from build123d import *

# Parameters (mm, degrees)
F1_DEPTH = 152.4
F3_DEPTH = 149.225
F5_DEPTH = 25.4


with BuildPart() as f1:
    # F0 (on Top) → F1 (new body)
    with BuildSketch(Plane.XY):
        Polygon((-177.8, 774.7), (-190.5, 0), (190.5, 0), (177.8, 774.7), align=None)
        Polygon((190.5, 0), (-190.5, 0), (0, -31.75), align=None)
    extrude(amount=F1_DEPTH)

    # F2 (on face) → F3 (cut)
    with BuildSketch(Plane(origin=(0, 0, 0), x_dir=(1, 0, 0), z_dir=(0, 0, -1))):
        Polygon((0, 28.5312048277), (-180.9470539995, -1.6266375055), (-168.3257693684, -771.525), (168.3257693684, -771.525), (180.9470539995, -1.6266375055), align=None)
    extrude(amount=-F3_DEPTH, mode=Mode.SUBTRACT)

    # F4 (on face) → F5 (cut)
    with BuildSketch(Plane.XY.offset(152.4)):
        with BuildLine():
            Line((114.3, 717.55), (-114.3, 717.55))
            ThreePointArc((-114.3, 717.55), (-132.2605122421, 710.1105122421), (-139.7, 692.15))
            Line((-139.7, 692.15), (-139.7, 323.85))
            ThreePointArc((-139.7, 323.85), (-132.2605122421, 305.8894877579), (-114.3, 298.45))
            Line((-114.3, 298.45), (114.3, 298.45))
            ThreePointArc((114.3, 298.45), (132.2605122421, 305.8894877579), (139.7, 323.85))
            Line((139.7, 323.85), (139.7, 692.15))
            ThreePointArc((139.7, 692.15), (132.2605122421, 710.1105122421), (114.3, 717.55))
        make_face()
    extrude(amount=-F5_DEPTH, mode=Mode.SUBTRACT)


solid = f1.part
The listing builds one solid part. Answer for the finished solid, in the listing's coordinates (mm). A direction names the side the tool comes from. Round coordinates to 2 decimals unless told otherwise and drop trailing zeros. Loops run counter-clockwise (first coordinate to the right, second up) from the corner with the lowest first, then second, coordinate; pieces in that order, holes last. Notation, with made-up numbers: M -21.75,46.25 L -15.75,46.25 A10 ccw -15.75,56.25 Z; hole C 34.5,-31.5 d6. An arc over 180 degrees is marked long. Write each question's results on one line, items separated by ' | '. Start each with the question number.
1) Find section B-B on x = 12.5. Write down the section's boundary in (y, z) (3 decimals), plus the area to 3 significant figures.
2) Which of the six approach directions +Z, -Z, +X, -X, +Y, -Y give full straight-line access (tool end or side, diameter ignored) to faces 5 (the flat face through (-3, 288, 152.4)), 6 (the flat face through (-2, 771.525, 74)), 7 (the cylindrical face through (-132.46, 306.09, 150.83))?
3) Straight lines are drawn through the part: probe 1 along Y at (x, z) = (-0.5, 111) (3 decimals); probe 2 along X at (y, z) = (416, 100); probe 3 along Y at (x, z) = (77.5, 119) (3 decimals). For each, find the intervals that lie inside material, in ascending order.
4) Find section D-D on x = 154. Write down the section's boundary in (y, z) (3 decimals), plus the area to 3 significant figures.
5) Determine the mould class of faces 1 (the flat face through (-3, 277, 149.225)), 2 (the cylindrical face through (132.06, 305.69, 150.83)), 3 (the flat face through (-96.583, -15.653, 75.133)), 4 (the flat face through (2, 774.7, 75)) for opening direction Y: pulls with the +Y half, pulls with the -Y half, needs draft (parallel to the pull), parting line crosses it, or undercut.
6) Find section C-C on y = 663.5. Write down the section's boundary in (x, z) (3 decimals), plus the area to 3 significant figures.
7) Each of these flat-tipped pins is pushed along its axis until it touches: pin 1 (2.5 mm diameter, centred on y = 514.5, z = 151, fed in from -X); pin 2 (1 mm diameter, centred on x = -43.5, z = 20.5, fed in from -Y); pin 3 (1 mm diameter, centred on y = 485.5, z = 151, fed in from +X). Where does it stop, or does it pass through?
8) Find section A-A on z = 47. Write down the section's boundary in (x, y) (3 decimals), plus the area to 3 significant figures.
Final values:
1) outline: M -29.667,0 L -26.448,0 L -26.448,149.225 L 298.45,149.225 L 298.45,152.4 L -29.667,152.4 Z; M 717.55,149.225 L 771.525,149.225 L 771.525,0 L 774.7,0 L 774.7,152.4 L 717.55,152.4 Z | area: 2,180 mm²
2) face 5: +Z, +X, -X, +Y, -Y | face 6: -Z | face 7: +Z, -Z
3) probe 1: -31.667 to -28.448, 771.525 to 774.7 | probe 2: -183.68 to -174.15, 174.15 to 183.68 | probe 3: -18.833 to -15.615, 771.525 to 774.7
4) outline: M -6.083,0 L -2.865,0 L -2.865,149.225 L 771.525,149.225 L 771.525,0 L 774.7,0 L 774.7,152.4 L -6.083,152.4 Z | area: 3,430 mm²
5) face 1: undercut | face 2: undercut | face 3: pulls with the -Y half | face 4: pulls with the +Y half
6) outline: M -179.623,0 L -170.097,0 L -170.097,149.225 L -139.7,149.225 L -139.7,152.4 L -179.623,152.4 Z; M 139.7,149.225 L 170.097,149.225 L 170.097,0 L 179.623,0 L 179.623,152.4 L 139.7,152.4 Z | area: 3,100 mm²
7) pin 1: x = -182.09 | pin 2: y = -24.58 | pin 3: x = 182.55
8) outline: M -190.5,0 L 0,-31.75 L 190.5,0 L 177.8,774.7 L -177.8,774.7 Z; hole M -180.947,1.627 L 0,-28.531 L 180.947,1.627 L 168.326,771.525 L -168.326,771.525 Z | area: 17,000 mm²
